Input: part model. Units: mm. Frame: model coordinates. Face numbers are marked on the shaded views. A direction names the side the tool comes from. Round coordinates to 2 decimals unless told otherwise and drop trailing zeros. Loops run counter-clockwise (first coordinate to the right, second up) from the corner with the lowest first, then second, coordinate; pieces in that order, holes last. Notation, with made-up numbers: M 32,53 L 80,53 A10 ccw 80,69 Z; hole C -29.5,16 d10. An arc over 180 degrees is marked long. Return JSON: item names as keys, results as strings. Group by question number.
1) Material intervals for line 1 (X direction, y = -22.5, z = 0.25); line 2 (X direction, y = 6.5, z = -1.5); line 3 (Y direction, x = 70, z = 0.25), sorted ascending. Write a range as from..to.
2) Access query for the marked faces 5, 6, 7 and 8. Directions: +Z, -Z, +X, -X, +Y, -Y. A direction counts if a zero-diameter tool reaches every point of the face in a straight line with its end or side. Return the directions, or none.
3) Contact query for flat-ended pins moving along their axis: P1, Ø5.5, axis at x = 14, z = -3, coming from the +Y side; P2, Ø6, axis at y = -7, z = 3.5, coming from the -X side; P3, Ø3.5, axis at x = 75, z = 2.5, coming from the +Y side; P4, Ø1.5, axis at x = 50, y = 10.5, coming from the +Z side. Output: stop coordinate, or through.
4) Section C-C (x = 9). Output: boundary loops of the cut face in (y, z) (3 decimals).
5) Mould query, pull axis Y, two halves, no side actions, for the marked faces 1, 2, 3 and 4. Classes: +Y half, -Y half, draft (parallel to the pull), parting line (faces both ways), or undercut.
6) Section B-B (x = 75.5). Output: boundary loops of the cut face in (y, z).
7) Section D-D (z = 0). Count the separate pieces of the cut face and the enclosed holes in it, plus the area to 3 significant figures.
8) Section A-A (y = -28). Output: boundary loops of the cut face in (x, z), plus the area to 3 significant figures.
from build123d import *

# Parameters (mm, degrees)
SKETCH1_W                = 96.52
SKETCH1_H                = 44.45
BOSS_EXTRUDE1_DEPTH      = 6.096
CUT_EXTRUDE1_REACH       = 108.961
SKETCH2_R                = 11.50874
CUT_EXTRUDE2_REACH       = 108.438
SKETCH3_R                = 3.3782
CUT_EXTRUDE3_REACH       = 108.961
SKETCH7_W                = 12.7635
SKETCH7_H                = 12.192
CUT_EXTRUDE5_DEPTH       = 104.946532487
FILLET1_R                = 11.43
CUT_EXTRUDE9_REACH       = 97.016
CUT_EXTRUDE9_END_RADIUS  = 11.50874
SKETCH11_R               = 2.0193
BOSS_EXTRUDE2_DEPTH      = 6.096
FILLET2_R                = 3.175
FILLET3_R                = 12.7
FILLET4_R                = 9.525
CUT_EXTRUDE10_DEPTH      = 57.546170308
CUT_EXTRUDE10_DEPTH_BACK = 57.546170308
SKETCH15_R               = 3.3782


with BuildPart() as part:
    # Sketch1 → Boss-Extrude1 (new, symmetric)
    with BuildSketch(Plane.XY):
        with Locations((48.26, -22.225)):
            Rectangle(SKETCH1_W, SKETCH1_H)
    extrude(amount=BOSS_EXTRUDE1_DEPTH, both=True)

    # Sketch2 → Cut-Extrude1 (cut, up to next)
    with BuildSketch(Plane.XY.offset(6.096), mode=Mode.PRIVATE) as cut_extrude1_sk1:
        with Locations((22.225, -22.225)):
            Circle(SKETCH2_R)
    cut_extrude1_tool1 = extrude(cut_extrude1_sk1.sketch, amount=-CUT_EXTRUDE1_REACH, mode=Mode.PRIVATE) & part.part
    add(cut_extrude1_tool1.solids().sort_by_distance((22.225, -22.225, 6.096))[0], mode=Mode.SUBTRACT)

    # Sketch3 → Cut-Extrude2 (cut, up to next)
    with BuildSketch(Plane(origin=(0, 0, 0), x_dir=(1, 0, 0), z_dir=(0, 1, 0)), mode=Mode.PRIVATE) as cut_extrude2_sk1:
        with Locations(Location((77.4065, -0.254, 0), (0, 0, 270))):
            Circle(SKETCH3_R)
    cut_extrude2_tool1 = extrude(cut_extrude2_sk1.sketch, amount=-CUT_EXTRUDE2_REACH, mode=Mode.PRIVATE) & part.part
    add(cut_extrude2_tool1.solids().sort_by_distance((77.4065, 0, 0.254))[0], mode=Mode.SUBTRACT)

    # Sketch4 → Cut-Extrude3 (cut, up to next)
    with BuildSketch(Plane.XY.offset(6.096), mode=Mode.PRIVATE) as cut_extrude3_sk1:
        with BuildLine():
            Line((48.895, 6.35), (96.52, 6.35))
            ThreePointArc((96.52, 6.35), (102.87, 0), (96.52, -6.35))
            Line((96.52, -6.35), (48.895, -6.35))
            ThreePointArc((48.895, -6.35), (42.545, 0), (48.895, 6.35))
        make_face()
    cut_extrude3_tool1 = extrude(cut_extrude3_sk1.sketch, amount=-CUT_EXTRUDE3_REACH, mode=Mode.PRIVATE) & part.part
    # Sketch4 → Cut-Extrude3 (cut, up to next)
    with BuildSketch(Plane.XY.offset(6.096), mode=Mode.PRIVATE) as cut_extrude3_sk2:
        with BuildLine():
            Line((45.72, -34.925), (45.72, -44.45))
            Line((45.72, -44.45), (55.245, -44.45))
            Line((55.245, -44.45), (96.52, -44.45))
            ThreePointArc((96.52, -44.45), (106.045, -34.925), (96.52, -25.4))
            Line((96.52, -25.4), (55.245, -25.4))
            ThreePointArc((55.245, -25.4), (48.509807909, -28.189807909), (45.72, -34.925))
        make_face()
    cut_extrude3_tool2 = extrude(cut_extrude3_sk2.sketch, amount=-CUT_EXTRUDE3_REACH, mode=Mode.PRIVATE) & part.part
    add(cut_extrude3_tool1.solids().sort_by_distance((72.7075, 0, 6.096))[0], mode=Mode.SUBTRACT)
    add(cut_extrude3_tool2.solids().sort_by_distance((75.382091, -35.05704, 6.096))[0], mode=Mode.SUBTRACT)

    # Sketch7 → Cut-Extrude5 (cut, through all)
    with BuildSketch(Plane(origin=(0, -6.35, 0), x_dir=(1, 0, 0), z_dir=(0, 1, 0))):
        with Locations((90.13825, 0)):
            Rectangle(SKETCH7_W, SKETCH7_H)
    extrude(amount=-CUT_EXTRUDE5_DEPTH, mode=Mode.SUBTRACT)

    # Fillet1
    fillet1_edges = [part.edges().sort_by_distance(p)[0] for p in [
        (42.545, 0, 0),
        (45.72, -44.45, 0),
        (0, -44.45, 0),
        (0, 0, 0),
    ]]
    fillet(fillet1_edges, radius=FILLET1_R)

    # Cut-Extrude9: up to this cylinder (the profile starts outside it)
    cut_extrude9_end = Plane(origin=(22.225, -22.225, 0), z_dir=(0, 0, 1)) * Cylinder(CUT_EXTRUDE9_END_RADIUS, 218.04948, mode=Mode.PRIVATE)
    # Sketch11 → Cut-Extrude9 (cut, up to the surface)
    with BuildSketch(Plane.ZY, mode=Mode.PRIVATE) as cut_extrude9_sk1:
        with Locations(Location((0, -22.225, 0), (0, 0, 270))):
            Circle(SKETCH11_R)
    cut_extrude9_tool1 = extrude(cut_extrude9_sk1.sketch, amount=-CUT_EXTRUDE9_REACH, mode=Mode.PRIVATE) - cut_extrude9_end
    add(cut_extrude9_tool1.solids().sort_by_distance((0, -22.225, 0))[0], mode=Mode.SUBTRACT)

    # Sketch14 → Boss-Extrude2 (add, symmetric)
    with BuildSketch(Plane.XY):
        Polygon((45.045272578, -5.496900798), (51.619276324, 19.03761519), (45.485647327, 20.681116126), (38.911643582, -3.853399862), align=None)
        Polygon((26.270231172, 0), (32.844234917, 0), (38.86132801, 22.456097137), (32.727699014, 24.099598074), align=None)
    extrude(amount=BOSS_EXTRUDE2_DEPTH, both=True)

    # Fillet2
    fillet2_edges = [part.edges().sort_by_distance(p)[0] for p in [
        (32.844234917, 0, 0),
        (39.704874489, -0.893021814, 0),
    ]]
    fillet(fillet2_edges, radius=FILLET2_R)

    # Fillet3
    fillet3_edges = [part.edges().sort_by_distance(p)[0] for p in [
        (26.270231172, 0, 0),
    ]]
    fillet(fillet3_edges, radius=FILLET3_R)

    # Fillet4
    fillet4_edges = [part.edges().sort_by_distance(p)[0] for p in [
        (45.14505865, -5.124494109, 0),
    ]]
    fillet(fillet4_edges, radius=FILLET4_R)

    # Sketch15 → Cut-Extrude10 (cut, two sides: drawn at the far end of the back side and taken through both)
    with BuildSketch(Plane(origin=(43.402036675, -11.629540677, 0), x_dir=(0, 0, -1), z_dir=(0.9659258262890672, -0.25881904510252485, 0)).offset(-CUT_EXTRUDE10_DEPTH_BACK)):
        with Locations(Location((0, 24.80969599, 0), (0, 0, 90))):
            Circle(SKETCH15_R)
    extrude(amount=CUT_EXTRUDE10_DEPTH + CUT_EXTRUDE10_DEPTH_BACK, mode=Mode.SUBTRACT)


solid = part.part
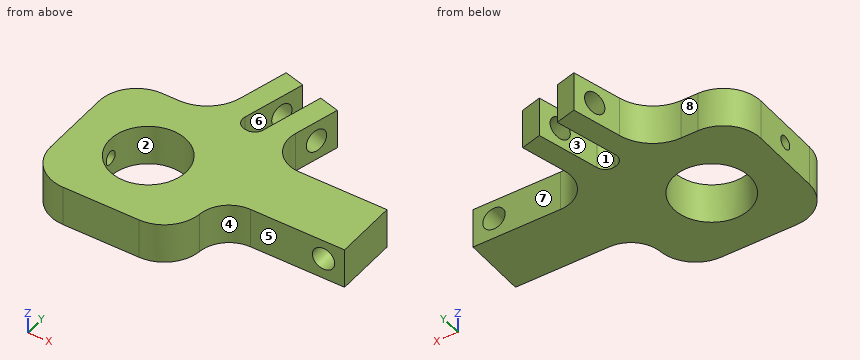
Returned:
{
 "1": {"line 1": "x = 33.73..74.03, 80.78..83.76", "line 2": "x = 27.61..34.59, 41.69..48.26", "line 3": "y = -25.4..-6.35"},
 "2": {"face 5": "+Z, -Z, +X, -Y", "face 6": "+Z, -Z", "face 7": "+Z, -Z, +X, +Y", "face 8": "+Z, -Z, -X, +Y"},
 "3": {"P1": "stops at y = 0", "P2": "stops at x = 0.09", "P3": "stops at y = -6.35", "P4": "stops at z = 6.1"},
 "4": {"outline": "M -44.189,-6.096 L -0.261,-6.096 L -0.261,6.096 L -44.189,6.096 Z; hole C -22.225,0 d4.039"},
 "5": {"face 1": "undercut", "face 2": "undercut", "face 3": "+Y half", "face 4": "-Y half"},
 "6": {"outline": "M -25.4,-6.1 L -6.35,-6.1 L -6.35,-2.53 L -25.4,-2.53 Z; M -25.4,3.04 L -6.35,3.04 L -6.35,6.1 L -25.4,6.1 Z"},
 "7": {"separate pieces": "4", "enclosed holes": "0", "area": "2,360 mm^2"},
 "8": {"outline": "M 0,-6.1 L 12.27,-6.1 L 12.27,6.1 L 0,6.1 Z; M 32.18,-6.1 L 48.71,-6.1 L 48.71,6.1 L 32.18,6.1 Z", "area": "351 mm^2"}
}
